Can you work these out from the drawing? Everything is in mm from the part's minimum corner. A direction names the side the tool comes from. Give positions to 0.01 mm unless a question says otherwise; leave off trailing zeros. Loops run counter-clockwise (first coordinate to the right, second up) from the corner with the lowest first, then second, coordinate; pieces in that order, holes last.
Q1. We'd pull the mould along Z, two halves only. Please class the marked faces 1, 2 and 3: +Z half, -Z half, draft (parallel to the pull), parting line (faces both ways), or undercut.
Q2. For the marked faces 4 and 5, which set-ups out of +Z, -Z, +X, -X, +Y, -Y let a thin tool reach every point of the face, with its end or its side?
Q3. If we section it at B-B (y = 43.5): Please give me the cut outline in (x, z) (1 decimal), plus the area to 3 significant figures.
Q4. If we section it at A-A (y = 23.5): Please give me the cut outline in (x, z) (1 decimal), plus the area to 3 significant figures.
Q5. Will these pins go through, and if not, where does the flat tip stop? P1, Ø1.5, axis at x = 29, y = 19.5, coming from the -Z side; P2, Ø12, axis at x = 89, y = 28, coming from the -Z side; P3, Ø12, axis at x = 27.5, z = 18.5, coming from the +Y side.
Q6. I need wall thicknesses on line 1 (Z direction, x = 56, y = 54.5) (1 decimal); line 2 (Z direction, x = 55.5, y = 47) (1 decimal); line 3 (X direction, y = 10, z = 57). Which ranges of each line are inside material? Lowest first, please.
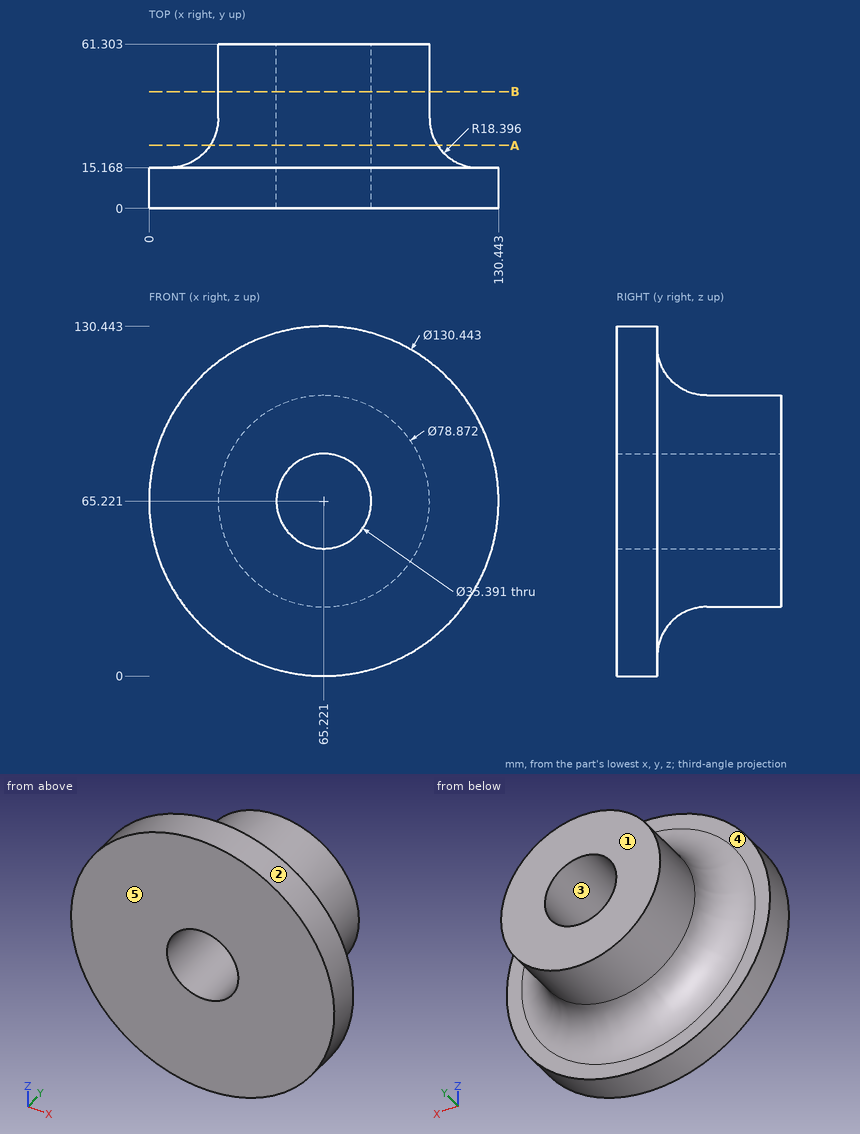
Check sheet entries:
1. face 1: draft
1. face 2: parting line
1. face 3: undercut
2. face 4: +Y
2. face 5: +Z, -Z, +X, -X, -Y
3. outline: circle Ø78.9 at (65.2, 65.2); hole circle Ø35.4 at (65.2, 65.2)
3. area: 3,900 mm2
4. outline: circle Ø84.9 at (65.2, 65.2); hole circle Ø35.4 at (65.2, 65.2)
4. area: 4,670 mm2
5. P1: stops at z = 35.15
5. P2: stops at z = 27.66
5. P3: stops at y = 15.56
6. line 1: z = 26.9 to 50.1, 80.3 to 103.6
6. line 2: z = 27 to 50.4, 80 to 103.4
6. line 3: x = 0.52 to 49.55, 80.89 to 129.92
